Geometry: final body of the model. Coordinates: model frame, mm. A direction names the side the tool comes from. Round coordinates to 2 decimals unless told otherwise and drop trailing zeros. Write each loop counter-clockwise with the first axis right and the second up, starting at its lowest first coordinate (ties: lowest second). Pieces come first, ordered by that corner, then holes. Notation, with made-up numbers: M -12,46 L 10,46 A24 cw 10,61 Z; hole C -0.5,50.5 d11. An arc over 180 degrees is marked long. Use one line per item in the form item = value. Start each with the question number.
from build123d import *

# Parameters (mm, degrees)
SKETCH1_W           = 18
SKETCH1_H           = 16
SKETCH1_R           = 5
BOSS_EXTRUDE2_DEPTH = 20
SKETCH3_R           = 1.605
CUT_EXTRUDE1_DEPTH  = 10
SKETCH4_R           = 1.6
CUT_EXTRUDE2_DEPTH  = 10
FILLET1_R           = 2


with BuildPart() as part:
    # Sketch1 → Boss-Extrude2 (new body)
    with BuildSketch(Plane(origin=(0, 0, 0), x_dir=(1, 0, 0), z_dir=(0, 1, 0))):
        with Locations((-15.037129634, 3.2340174)):
            Rectangle(SKETCH1_W, SKETCH1_H)
        with Locations(Location((-15.204317972, 3.2340174, 0), (0, 0, 270))):
            Circle(SKETCH1_R, mode=Mode.SUBTRACT)
    extrude(amount=BOSS_EXTRUDE2_DEPTH)

    # Sketch3 → Cut-Extrude1 (cut)
    with BuildSketch(Plane(origin=(-6.037129634, 0, 0), x_dir=(0, 0, -1), z_dir=(1, 0, 0))):
        with Locations((2.2340174, 10)):
            Circle(SKETCH3_R)
    extrude(amount=-CUT_EXTRUDE1_DEPTH, mode=Mode.SUBTRACT)

    # Sketch4 → Cut-Extrude2 (cut)
    with BuildSketch(Plane.XY.offset(4.7659826)):
        with Locations((-15.037129634, 10)):
            Circle(SKETCH4_R)
    extrude(amount=-CUT_EXTRUDE2_DEPTH, mode=Mode.SUBTRACT)

    # Fillet1
    fillet1_edges = [part.edges().sort_by_distance(p)[0] for p in [
        (-6.037129634, 10, 4.7659826),
    ]]
    fillet(fillet1_edges, radius=FILLET1_R)


solid = part.part
1. Set-up query: faces 1 (the face through (-6.639, 10.14, 4.196)), 2 (the face through (-8.46, 10.07, -0.63)). Return all of +Z, -Z, +X, -X, +Y, -Y with unobstructed straight access to the full face (end or side cutting, diameter ignored); none if empty.
2. Section query B-B (y = 10). Return loops of the section in (x, z), then the cut area to 3 significant figures.
3. Pull-direction query (X, two-part tool) for faces 3 (the face through (-24.037, 10, -3)), 4 (the face through (-15.384, 8.438, 3.128)), 5 (the face through (-18, 10, 4.766)); classes: released by +X, released by -X, zero draft, split by the parting line, or undercut.
4. Ray query, probe 1 along Z at (x, y) = (-9.65, 10); probe 2 along Z at (x, y) = (-15, 12.75); probe 3 along X at (y, z) = (9.5, -5.5). Return the intervals inside material, ascending.
5. Section query A-A (x = -11.25). Return loops of the section in (y, z).
6. Section query D-D (x = -18.75). Return loops of the section in (y, z).
7. Section query C-C (y = 7). Return loops of the section in (x, z).
8. Contact query for flat-ended pins moving along their axis: pin 1 (1.5 mm diameter, centred on x = -15.5, z = -5.5, fed in from -Y); pin 2 (2.5 mm diameter, centred on x = -15.04, y = 10, fed in from +Z). Output: stop coordinate, or through.
Checks:
q1.face_1 = +Z, +X, +Y, -Y
q1.face_2 = +X
q2.outline = M -24.04,-11.23 L -6.04,-11.23 L -6.04,-3.84 L -10.24,-3.84 A5 cw long -16.64,1.56 L -16.64,4.77 L -24.04,4.77 Z; M -13.44,1.44 A5 cw -10.94,-0.63 L -6.04,-0.63 L -6.04,2.77 A2 ccw -8.04,4.77 L -13.44,4.77 Z
q2.area = 185 mm^2
q3.face_3 = released by -X
q3.face_4 = undercut
q3.face_5 = zero draft
q4.probe_1 = -11.23 to -3.84, -0.63 to 4.77
q4.probe_2 = -11.23 to -8.23, 1.76 to 4.77
q4.probe_3 = -24.04 to -19.66, -10.75 to -6.04
q5.outline = M 0,-11.23 L 20,-11.23 L 20,-6.29 L 0,-6.29 Z; M 0,-0.17 L 20,-0.17 L 20,4.77 L 0,4.77 Z
q6.outline = M 0,-11.23 L 20,-11.23 L 20,-6.76 L 0,-6.76 Z; M 0,0.29 L 20,0.29 L 20,4.77 L 0,4.77 Z
q7.outline = M -24.04,-11.23 L -6.04,-11.23 L -6.04,2.77 A2 ccw -8.04,4.77 L -24.04,4.77 Z; hole C -15.2,-3.23 d10
q8.pin_1 = through
q8.pin_2 = -8.03
